For this review, take the finished solid that the model builds, in its own axes (mm). Round coordinates to 2 decimals unless told otherwise and drop trailing zeros. Write each loop counter-clockwise with the first axis right and the second up, starting at its lowest first coordinate (ties: lowest second). Pieces come first, ordered by that corner, then holes. Notation, with made-up numbers: (69.5, -4.75) - (94.5, -4.75) arc R28 cw to (94.5, 29.25) - close; hole circle Ø2 at (30, 12). An arc over 180 degrees is marked (long way). One line per item, written item: value. Start each with the question number.
Q1. Add section A-A on z = -10. Write out the cut boundary in (x, y), and give its area (3 significant figures).
Q2. Clearance check with flat-ended pins moving along their axes: pin 1 Ø2 at (x, y) = (8, 14.5) entering from -Z; pin 2 Ø3.5 at (y, z) = (7.93, 43.73) entering from +X. State where each tip first meets the part, or that it passes through.
Q3. Add section B-B on x = -11.5. Give the number of separate pieces and of enclosed holes in the cut face, and give its area (3 significant figures).
Q4. For probe 1 along Y at (x, z) = (8, -49); probe 2 along Z at (x, y) = (-3.5, 11.25); probe 3 along Y at (x, z) = (8, -42.4), list the stretches that pass through material, from the lowest coordinate up.
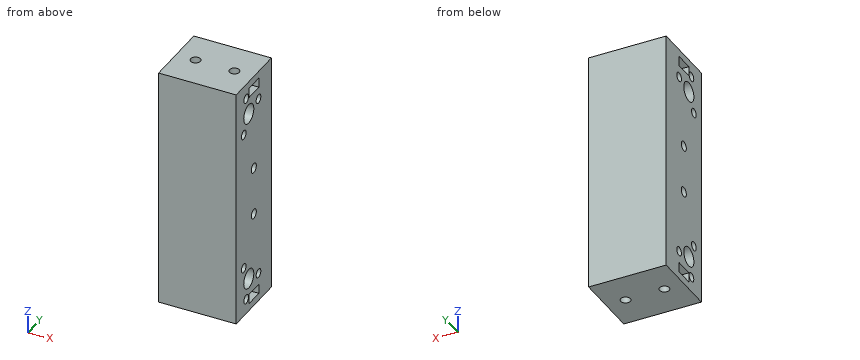
Autodesk Inventor part; units mm, degrees
ref_plane "РабПлоскость1" through (-16, 0, 47) normal (0, 0, 1) x (1, 0, 0)
ref_plane "YZ Plane" through (0, 0, 0) normal (1, 0, 0) x (0, 1, 0)
ref_plane "XZ Plane" through (0, 0, 0) normal (0, 1, 0) x (-1, 0, 0)
sketch "Эскиз1" plane through (0, 0, 0) normal (0, 1, 0) x (-1, 0, 0)
  line L0 (-16, 50) -> (16, 50)
  line L1 (16, 50) -> (16, -50)
  line L2 (16, -50) -> (-16, -50)
  line L3 (-16, -50) -> (-16, 50)
  line L4 (-16, 50) -> (16, -50) construction
  line L5 (16, 50) -> (-16, -50) construction
  point P0 (0, 0)
  dimension "d0" = 32
  dimension "d1" = 100
extrude "Выдавливание1" add sketch "Эскиз1" along normal blind 28
sketch "Эскиз2" plane through (16, 0, 50) normal (1, 0, 0) x (0, 0, -1)
  circle A0 centre (86, 10) radius 4
  line L0 (100, 0) -> (100, 28)
  line L1 (0, 0) -> (100, 0)
  point P0 (50, 0)
  dimension "d4" = 8
  dimension "d5" = 14
  dimension "d6" = 10
extrude "Выдавливание2" cut sketch "Эскиз2" against normal through all
mirror "Зеркальное отражение1" about plane through (0, 0, 0) normal (0, 0, 1) of "Выдавливание2"
sketch "Эскиз3" plane through (16, 0, 50) normal (1, 0, 0) x (0, 0, -1)
  circle A0 centre (11.9294, 17.7274) radius 1.85
  circle A1 centre (20.9282, 6) radius 1.85
  circle A2 centre (79.0718, 6) radius 1.85
  circle A3 centre (88.0706, 17.7274) radius 1.85
  circle A4 centre (93.7274, 7.9294) radius 1.85
  circle A5 centre (6.2726, 7.9294) radius 1.85
  point P0 (50, 0)
extrude "Выдавливание3" cut sketch "Эскиз3" against normal through all
sketch "Эскиз4" plane through (16, 0, 50) normal (1, 0, 0) x (0, 0, -1)
  line L0 (50, 0) -> (50, 14) construction
  line L1 (50, 14) -> (40, 14) construction
  circle A0 centre (40, 14) radius 2
  dimension "d11" = 10
  dimension "d12" = 14
  dimension "d13" = 4
extrude "Выдавливание4" cut sketch "Эскиз4" against normal through all
mirror "Зеркальное отражение2" about plane through (0, 0, 0) normal (0, 0, 1) of "Выдавливание4"
sketch "Эскиз5" plane through (-16, 0, 50) normal (0, 0, 1) x (1, 0, 0)
  circle A0 centre (8, 14) radius 2
  line L0 (0, 0) -> (32, 0)
  line L1 (0, 0) -> (0, 28)
  point P0 (16, 0)
  dimension "d16" = 4
  dimension "d17" = 14
  dimension "d18" = 8
extrude "Выдавливание5" cut sketch "Эскиз5" against normal blind 8
ref_plane "РабПлоскость1" through (-16, 0, 47) normal (0, 0, 1) x (1, 0, 0)
sketch "Эскиз6" plane through (-16, 0, 47) normal (0, 0, 1) x (1, 0, 0)
  circle A0 centre (8, 14) radius 2
  line L0 (10.3094, 10) -> (5.6906, 10)
  line L1 (5.6906, 10) -> (3.3812, 14)
  line L2 (3.3812, 14) -> (5.6906, 18)
  line L3 (5.6906, 18) -> (10.3094, 18)
  line L4 (10.3094, 18) -> (12.6188, 14)
  line L5 (12.6188, 14) -> (10.3094, 10)
  line L6 (32, 0) -> (0, 0)
  line L7 (5.6906, 18) -> (0, 18)
  line L8 (32, 19.5774) -> (0, 19.5774)
  line L9 (5.6906, 10) -> (0, 10)
  line L10 (0, 6) -> (0, 14)
  line L11 (0, 18) -> (0, 10)
  point P0 (16, 0)
  point P1 (0, 14)
  dimension "d22" = 8
extrude "Выдавливание6" cut sketch "Эскиз6" against normal blind 4 contours A0 | L0 L1 L2 L3 L4 L5 | L9 L10 L11 L7 L2 L1
ref_plane "РабПлоскость2" through (0, 28, 50) normal (-1, 0, 0) x (0, 0, 1)
mirror "Зеркальное отражение3" about plane through (0, 28, 50) normal (-1, 0, 0) of "Выдавливание6", "Выдавливание5"
mirror "Зеркальное отражение4" about plane through (0, 0, 0) normal (0, 0, 1) of "Выдавливание6", "Выдавливание5", "Зеркальное отражение3"
properties part number "KB33-046-003-001 - Соединитель" material "Пластик АБС"
Result set:
1. outline: (-16, 0) - (16, 0) - (16, 12) - (-16, 12) - close; (-16, 16) - (16, 16) - (16, 28) - (-16, 28) - close
1. area: 768 mm^2
2. pin 1: stops at z = -42
2. pin 2: passes through
3. separate pieces: 1
3. enclosed holes: 12
3. area: 2,550 mm^2
4. probe 1: y = 0 to 12, 16 to 28
4. probe 2: z = -50 to -39.8, -32.2 to 32.2, 39.8 to 50
4. probe 3: y = 0 to 6.64, 9.22 to 12, 16 to 28
